For this review, use the dimensioned drawing (mm, ordinates from the lowest corner) and the shaded views. Round coordinates to 2 decimals unless told otherwise and drop trailing zeros. Loops run counter-clockwise (first coordinate to the right, second up) from the corner with the lowest first, then second, coordinate; pieces in that order, holes last. Notation, with made-up numbers: M 78.5,-10 L 132.5,-10 A24 ccw 132.5,22 Z; hole C 45.5,31 d5. An arc over 180 degrees is marked long. Answer as a JSON object with one key per item and string values. Group by question number.
Item 1: Consider section A-A (y = 7.75). Give the boundary of the cut face in (x, z).
Item 2: Consider section C-C (x = 56). Give the boundary of the cut face in (y, z), and give its area (3 significant figures).
Item 3: To check wall thickness, follow line 1 (X direction, y = 9.75, z = 52); line 2 (Z direction, x = 4, y = 8.5) (1 decimal); line 3 (X direction, y = 3.5, z = 36). State the ranges of each line that lie inside material, in increasing order.
Item 4: Consider section B-B (z = 14.5). Give the boundary of the cut face in (x, y).
Item 5: Insertion check: P1, Ø1, axis at x = 67, y = 4.5, coming from the -Z side (1 decimal); P2, Ø6, axis at x = 68.5, z = 22.5, coming from the +Y side. Each pin has a flat end and moves straight along its axis. Give the tip position at first contact, or say it passes through.
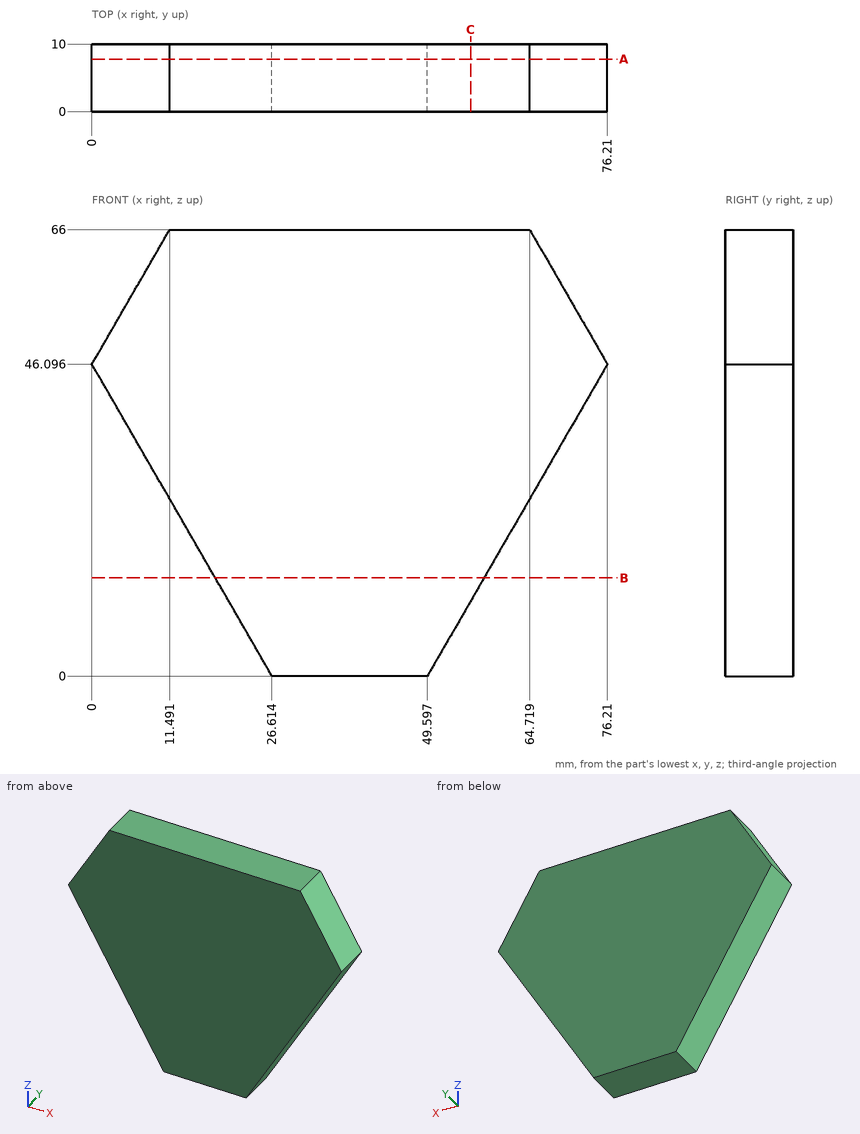
Geometry results:
{
 "1": {"outline": "M 0,46.1 L 26.61,0 L 49.6,0 L 76.21,46.1 L 64.72,66 L 11.49,66 Z"},
 "2": {"outline": "M 0,11.09 L 10,11.09 L 10,66 L 0,66 Z", "area": "549 mm^2"},
 "3": {"line 1": "x = 3.41 to 72.8", "line 2": "z = 39.2 to 53", "line 3": "x = 5.83 to 70.38"},
 "4": {"outline": "M 18.24,0 L 57.97,0 L 57.97,10 L 18.24,10 Z"},
 "5": {"P1": "stops at z = 29.3", "P2": "passes through"}
}
